from build123d import *

# Parameters (mm, degrees)
SKETCH1_W               = 381
SKETCH1_H               = 6.35
BASE_FLANGE1_DEPTH      = 831.85
CUT_EXTRUDE1_DEPTH      = 915.973084304
CUT_EXTRUDE1_DEPTH_BACK = 6.35
SKETCH9_R               = 3.429
CUT_EXTRUDE2_DEPTH      = 6.35
SKETCH10_R              = 3.429
CUT_EXTRUDE3_DEPTH      = 6.35
SKETCH11_W              = 101.6
SKETCH11_H              = 609.6
CUT_EXTRUDE4_DEPTH      = 6.35
BOSS_EXTRUDE1_START     = -6.35
BOSS_EXTRUDE1_DEPTH     = 6.35


# Sheet-metal steps are written as plain solids
with BuildPart() as part:
    # Sketch1 → Base-Flange1 (new body)
    with BuildSketch(Plane.XY):
        with Locations((190.5, -3.175)):
            Rectangle(SKETCH1_W, SKETCH1_H)
    extrude(amount=BASE_FLANGE1_DEPTH)

    # Sketch8 → Cut-Extrude1 (cut, two sides: drawn at the far end of the back side and taken through both)
    with BuildSketch(Plane(origin=(0, 0, 0), x_dir=(1, 0, 0), z_dir=(0, 1, 0)).offset(-CUT_EXTRUDE1_DEPTH_BACK)):
        Polygon((381, -672.879100114), (0, -831.85), (381, -831.85), align=None)
    extrude(amount=CUT_EXTRUDE1_DEPTH + CUT_EXTRUDE1_DEPTH_BACK, mode=Mode.SUBTRACT)

    # Sketch9 → Cut-Extrude2 (cut)
    with BuildSketch(Plane(origin=(0, 0, 0), x_dir=(1, 0, 0), z_dir=(0, 1, 0))):
        with Locations(Location((130.175, -12.7, 0), (0, 0, 270))):
            Circle(SKETCH9_R)
        with Locations(Location((53.975, -12.7, 0), (0, 0, 270))):
            Circle(SKETCH9_R)
    extrude(amount=-CUT_EXTRUDE2_DEPTH, mode=Mode.SUBTRACT)

    # Sketch10 → Cut-Extrude3 (cut)
    with BuildSketch(Plane(origin=(0, 0, 0), x_dir=(1, 0, 0), z_dir=(0, 1, 0))):
        with Locations(Location((50.8, -796.892712954, 0), (0, 0, 270))):
            Circle(SKETCH10_R)
        with Locations(Location((121.123977295, -767.550282628, 0), (0, 0, 270))):
            Circle(SKETCH10_R)
        with Locations(Location((285.21325765, -699.084611868, 0), (0, 0, 270))):
            Circle(SKETCH10_R)
        with Locations(Location((355.537234945, -669.742181542, 0), (0, 0, 270))):
            Circle(SKETCH10_R)
        with Locations(Location((260.35, -12.7, 0), (0, 0, 270))):
            Circle(SKETCH10_R)
        with Locations(Location((336.55, -12.7, 0), (0, 0, 270))):
            Circle(SKETCH10_R)
    extrude(amount=-CUT_EXTRUDE3_DEPTH, mode=Mode.SUBTRACT)

    # Sketch11 → Cut-Extrude4 (cut)
    with BuildSketch(Plane(origin=(0, 0, 0), x_dir=(1, 0, 0), z_dir=(0, 1, 0))):
        with Locations((241.3, -355.6)):
            Rectangle(SKETCH11_W, SKETCH11_H)
    extrude(amount=-CUT_EXTRUDE4_DEPTH, mode=Mode.SUBTRACT)

    # Sketch12 → Boss-Extrude1 (add)
    with BuildSketch(Plane(origin=(0, 0, 0), x_dir=(1, 0, 0), z_dir=(0, 1, 0)).offset(BOSS_EXTRUDE1_START)):
        Polygon((0, -831.85), (-152.4, -895.438359954), (-152.4, 0), (0, 0), align=None)
    extrude(amount=BOSS_EXTRUDE1_DEPTH)


solid = part.part
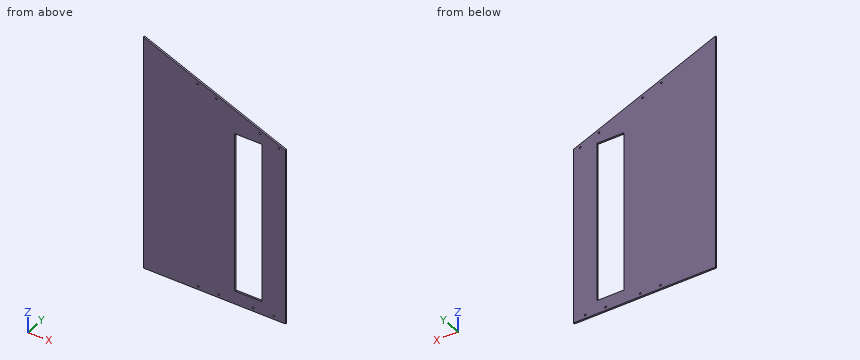
Can you work these out from the model? Positions are in its coordinate system, mm. Round coordinates to 2 decimals unless told otherwise and drop trailing zeros. Order: outer loops, then holes, each group sorted by start corner. A loop starts at its lowest first (then second) coordinate and runs counter-clockwise, first axis right, second up. Notation, with made-up numbers: M 84.5,16.5 L 105.5,16.5 A27 cw 105.5,45.5 Z; hole C 32.25,54 d1. An arc over 180 degrees is marked long. Use a Markdown table: item, result.
1) Imagine slicing it at D-D (z = 811.5). List the corners of the cut face in (x, y) for me.
Geometry says:
| item | result |
|---|---|
| outline | M -152.4,-6.35 L 48.77,-6.35 L 48.77,0 L -152.4,0 Z |
2) Imagine slicing it at B-B (x = 220). List the corners of the cut face in (y, z) for me, then the cut area to 3 significant figures.
Geometry says:
| item | result |
|---|---|
| outline | M -6.35,0 L 0,0 L 0,50.8 L -6.35,50.8 Z; M -6.35,660.4 L 0,660.4 L 0,740.06 L -6.35,740.06 Z |
| area | 828 mm² |
3) Imagine slicing it at C-C (y = -2.5). Give the number of separate pieces and of enclosed holes in the cut face, then the cut area to 3 significant figures.
Geometry says:
| item | result |
|---|---|
| separate pieces | 1 |
| enclosed holes | 9 |
| area | 356,000 mm² |
4) If I drill on line 1 along X through (y, z) = (-1.75, 12.7); line 2 along X through (y, z) = (-1.75, 482); line 3 along Z through (x, y) = (52, -1.25), over which ranges is the centre line in solid material (lowest first)?
Geometry says:
| item | result |
|---|---|
| line 1 | x = -152.4 to 50.55, 57.4 to 126.75, 133.6 to 256.92, 263.78 to 333.12, 339.98 to 381 |
| line 2 | x = -152.4 to 190.5, 292.1 to 381 |
| line 3 | z = 0 to 9.9, 15.5 to 793.68, 800.1 to 810.15 |
5) I'm going to push flat-ended pins straight in: P1, Ø5.5, axis at x = 53.975, z = 12.7, coming from the +Y side; P2, Ø3, axis at x = 147, y = -1.5, coming from the +Z side; P3, Ø1.5, axis at x = 12, y = -1.5, coming from the +Z side; P4, Ø1.9, axis at x = 259.5, y = -2, coming from the +Z side. Where does each tip first touch, or does it pass through?
Geometry says:
| item | result |
|---|---|
| P1 | passes through |
| P2 | stops at z = 771.14 |
| P3 | stops at z = 827.16 |
| P4 | stops at z = 723.97 |
6) Imagine slicing it at A-A (z = 298). List the corners of the cut face in (x, y) for me.
Geometry says:
| item | result |
|---|---|
| outline | M -152.4,-6.35 L 190.5,-6.35 L 190.5,0 L -152.4,0 Z; M 292.1,-6.35 L 381,-6.35 L 381,0 L 292.1,0 Z |
